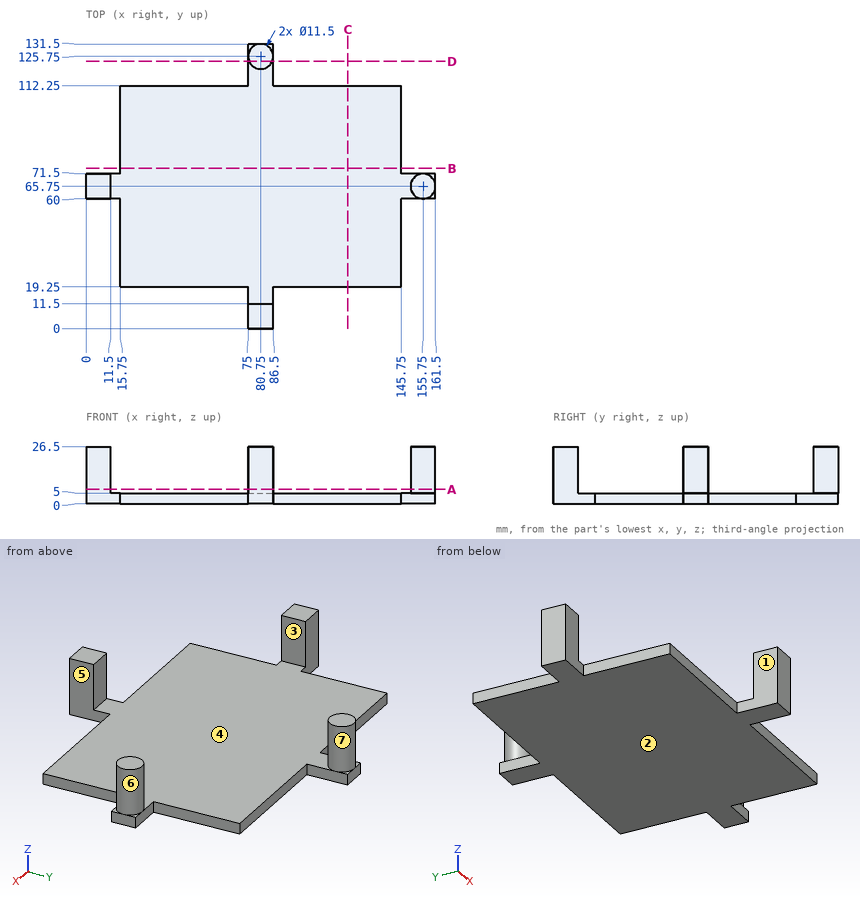
Part print with two shaded views. Sizes in mm from the minimum x, y, z corner. A direction names the side the tool comes from. Round coordinates to 2 decimals unless told otherwise and drop trailing zeros. Write each loop counter-clockwise with the first axis right and the second up, starting at its lowest first coordinate (ties: lowest second). Pieces come first, ordered by that corner, then holes. Notation, with made-up numbers: (18, 51) - (25, 51) arc R7 cw to (25, 60) - close; hole circle Ø5 at (61.25, 1). An arc over 180 degrees is marked (long way). Answer as CSV lines item,"result".
Q1. Tool access for the marked faces 1, 2, 3 and 4: list every direction of +Z, -Z, +X, -X, +Y, -Y with a clear straight run to the whole face (end or side of a thin tool).
Report:
face 1,"+Z, -Z, -X, -Y"
face 2,"-Z, +X, -X, +Y, -Y"
face 3,"+Z, +Y, -Y"
face 4,"+Z"
Q2. Cut at D-D (y = 123.5). Write the cut outline in (x, z).
Report:
outline,"(75, 0) - (86.5, 0) - (86.5, 5) - (86.04, 5) - (86.04, 26.5) - (75.46, 26.5) - (75.46, 5) - (75, 5) - close"
Q3. Cut at B-B (y = 74). Write the cut outline in (x, z), and give its area (3 significant figures).
Report:
outline,"(15.75, 0) - (145.75, 0) - (145.75, 5) - (15.75, 5) - close"
area,"650 mm^2"
Q4. Drop flat-ended pins along their axis: pin 1 (5.5 mm diameter, centred on y = 99, z = 3.5, fed in from -X); pin 2 (8 mm diameter, centred on y = 53.5, z = 23.5, fed in from +X) (1 decimal); pin 3 (1.5 mm diameter, centred on x = 157, z = 3.5, fed in from -Y); pin 4 (4 mm diameter, centred on y = 125.5, z = 1.5, fed in from -X). Give the stop position or say it passes through.
Report:
pin 1,"stops at x = 15.75"
pin 2,"passes through"
pin 3,"stops at y = 60"
pin 4,"stops at x = 75"
Q5. Drill centre lines: probe 1 along Z at (x, y) = (137.5, 36.5); probe 2 along Y at (x, z) = (24.5, 4); probe 3 along X at (y, z) = (68.5, 25). Where is each one in solid material? Low to high. Write a range as [from, to].
Report:
probe 1,"z = [0, 5]"
probe 2,"y = [19.25, 112.25]"
probe 3,"x = [0, 11.5], [150.7, 160.8]"
Q6. Cut at C-C (x = 121). Write the cut outline in (y, z), and give its area (3 significant figures).
Report:
outline,"(19.25, 0) - (112.25, 0) - (112.25, 5) - (19.25, 5) - close"
area,"465 mm^2"
Q7. Cut at A-A (z = 6.75). Write the cut outline in (x, y), and give its area (3 significant figures).
Report:
outline,"(0, 60) - (11.5, 60) - (11.5, 71.5) - (0, 71.5) - close; (75, 0) - (86.5, 0) - (86.5, 11.5) - (75, 11.5) - close; circle Ø11.5 at (80.75, 125.75); circle Ø11.5 at (155.75, 65.75)"
area,"472 mm^2"
Q8. Pull direction Y, two halves, no side cores. Call the marked faces 5, 6 and 7: +Y half, -Y half, draft (parallel to the pull), parting line (faces both ways), or undercut.
Report:
face 5,"draft"
face 6,"parting line"
face 7,"undercut"
